Here's how the part is built. I have some questions about the finished solid (model axes, mm). Round coordinates to 2 decimals unless told otherwise and drop trailing zeros. Loops run counter-clockwise (first coordinate to the right, second up) from the corner with the lowest first, then second, coordinate; pieces in that order, holes last. Notation, with made-up numbers: (69.25, 48.25) - (110.25, 48.25) arc R23 ccw to (110.25, 79.25) - close; hole circle Ø10 at (38.25, 46). An arc over 180 degrees is marked (long way). Answer as a JSON object with one key per item and string values. Group by question number.
1) I want a section at B-B, the plane z = 130. Please give me the cut outline in (x, y), then the cut area to 3 significant figures.
2) I want a section at A-A, the plane x = 25. Please give me the cut outline in (y, z).
3) I want a section at C-C, the plane z = 5. Please give me the cut outline in (x, y), then the cut area to 3 significant figures.
4) I want a section at D-D, the plane x = 12.5. Please give me the cut outline in (y, z), then the cut area to 3 significant figures.
5) Will these pins go through, and if not, where does the flat tip stop? P1, Ø5.5, axis at x = 29.5, z = 129, coming from the +Y side; P2, Ø11.5, axis at x = 25, z = 130, coming from the -Y side; P3, Ø5, axis at x = 37.5, z = 5, coming from the -Y side.
6) If I drill on line 1 along Z through (x, y) = (12.5, -13.8); line 2 along Z through (x, y) = (25, -1.25), over which ranges is the centre line in solid material (lowest first)? Write a range as [from, to].
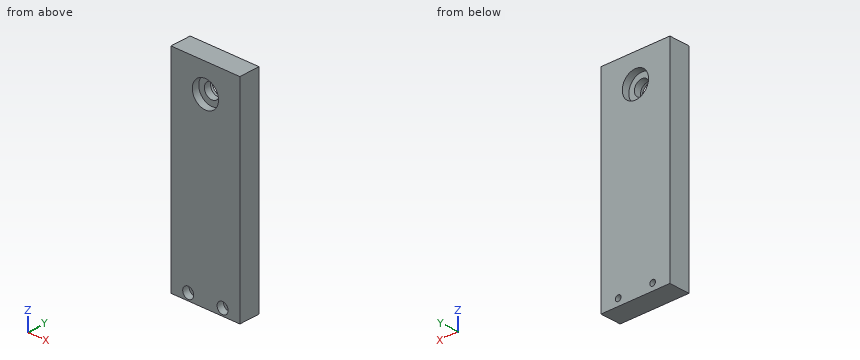
from build123d import *

# Parameters (mm, degrees)
F0_W     = 15
F0_H     = 150
F1_DEPTH = 50
F2_R     = 5.5
F2_R_2   = 2.05
F3_DEPTH = 15
F2_R_3   = 4
F4_DEPTH = 5
F2_R_4   = 9.55
F5_DEPTH = 5.1
F6_R     = 9.55
F6_R_2   = 5.5
F7_DEPTH = 5.1


with BuildPart() as f1:
    # F0 (on Right) → F1 (new body)
    with BuildSketch(Plane.YZ):
        with Locations((-7.5, 75)):
            Rectangle(F0_W, F0_H)
    extrude(amount=F1_DEPTH)

    # F2 (on face) → F3 (cut, through all)
    with BuildSketch(Plane.XZ.offset(15)):
        with Locations((25, 130)):
            Circle(F2_R)
        with Locations((12.5, 5)):
            Circle(F2_R_2)
        with Locations((37.5, 5)):
            Circle(F2_R_2)
    extrude(amount=-F3_DEPTH, mode=Mode.SUBTRACT)

    # F2 (on face) → F4 (cut)
    with BuildSketch(Plane.XZ.offset(15)):
        with Locations((12.5, 5)):
            Circle(F2_R_3)
        with Locations((12.5, 5)):
            Circle(F2_R_2, mode=Mode.SUBTRACT)
        with Locations((37.5, 5)):
            Circle(F2_R_3)
        with Locations((37.5, 5)):
            Circle(F2_R_2, mode=Mode.SUBTRACT)
    extrude(amount=-F4_DEPTH, mode=Mode.SUBTRACT)

    # F2 (on face) → F5 (cut)
    with BuildSketch(Plane.XZ.offset(15)):
        with Locations((25, 130)):
            Circle(F2_R_4)
        with Locations((25, 130)):
            Circle(F2_R, mode=Mode.SUBTRACT)
    extrude(amount=-F5_DEPTH, mode=Mode.SUBTRACT)

    # F6 (on face) → F7 (cut)
    with BuildSketch(Plane(origin=(0, 0, 0), x_dir=(-1, 0, 0), z_dir=(0, 1, 0))):
        with Locations((-25, 130)):
            Circle(F6_R)
        with Locations((-25, 130)):
            Circle(F6_R_2, mode=Mode.SUBTRACT)
    extrude(amount=-F7_DEPTH, mode=Mode.SUBTRACT)


solid = f1.part
Outcome:
{
 "1": {"outline": "(0, -15) - (15.45, -15) - (15.45, -9.9) - (19.5, -9.9) - (19.5, -5.1) - (15.45, -5.1) - (15.45, 0) - (0, 0) - close; (30.5, -9.9) - (34.55, -9.9) - (34.55, -15) - (50, -15) - (50, 0) - (34.55, 0) - (34.55, -5.1) - (30.5, -5.1) - close", "area": "502 mm^2"},
 "2": {"outline": "(-15, 0) - (0, 0) - (0, 120.45) - (-5.1, 120.45) - (-5.1, 124.5) - (-9.9, 124.5) - (-9.9, 120.45) - (-15, 120.45) - close; (-15, 139.55) - (-9.9, 139.55) - (-9.9, 135.5) - (-5.1, 135.5) - (-5.1, 139.55) - (0, 139.55) - (0, 150) - (-15, 150) - close"},
 "3": {"outline": "(0, -15) - (8.5, -15) - (8.5, -10) - (10.45, -10) - (10.45, 0) - (0, 0) - close; (14.55, -10) - (16.5, -10) - (16.5, -15) - (33.5, -15) - (33.5, -10) - (35.45, -10) - (35.45, 0) - (14.55, 0) - close; (39.55, -10) - (41.5, -10) - (41.5, -15) - (50, -15) - (50, 0) - (39.55, 0) - close", "area": "588 mm^2"},
 "4": {"outline": "(-15, 0) - (0, 0) - (0, 2.95) - (-10, 2.95) - (-10, 1) - (-15, 1) - close; (-15, 9) - (-10, 9) - (-10, 7.05) - (0, 7.05) - (0, 150) - (-15, 150) - close", "area": "2,170 mm^2"},
 "5": {"P1": "y = -5.1", "P2": "y = -9.9", "P3": "y = -10"},
 "6": {"line 1": "[0, 1], [9, 150]", "line 2": "[0, 120.45], [139.55, 150]"}
}
